from build123d import *

# Parameters (mm, degrees)
BOSS_EXTRUDE1_DEPTH = 40
SKETCH2_R           = 18
SKETCH2_R_2         = 1.5
BOSS_EXTRUDE2_DEPTH = 30.2
SKETCH3_R           = 11
BOSS_EXTRUDE3_DEPTH = 2
BOSS_EXTRUDE4_DEPTH = 20


with BuildPart() as part:
    # Sketch1 → Boss-Extrude1 (new body)
    with BuildSketch(Plane(origin=(0, 0, 0), x_dir=(0, 0, -1), z_dir=(1, 0, 0))):
        Polygon((-21, 15), (-15, 21), (15, 21), (21, 15), (21, -15), (15, -21), (-15, -21), (-21, -15), align=None)
    extrude(amount=BOSS_EXTRUDE1_DEPTH)

    # Sketch2 → Boss-Extrude2 (add)
    with BuildSketch(Plane(origin=(40, 0, 0), x_dir=(0, 0, -1), z_dir=(1, 0, 0))):
        Circle(SKETCH2_R)
        with Locations((-9.899494937, 9.899494937)):
            Circle(SKETCH2_R_2, mode=Mode.SUBTRACT)
        with Locations((9.899494937, 9.899494937)):
            Circle(SKETCH2_R_2, mode=Mode.SUBTRACT)
        with Locations((9.899494937, -9.899494937)):
            Circle(SKETCH2_R_2, mode=Mode.SUBTRACT)
        with Locations((-9.899494937, -9.899494937)):
            Circle(SKETCH2_R_2, mode=Mode.SUBTRACT)
    extrude(amount=BOSS_EXTRUDE2_DEPTH)

    # Sketch3 → Boss-Extrude3 (add)
    with BuildSketch(Plane(origin=(70.2, 0, 0), x_dir=(0, 0, -1), z_dir=(1, 0, 0))):
        Circle(SKETCH3_R)
    extrude(amount=BOSS_EXTRUDE3_DEPTH)

    # Sketch4 → Boss-Extrude4 (add)
    with BuildSketch(Plane(origin=(72.2, 0, 0), x_dir=(0, 0, -1), z_dir=(1, 0, 0))):
        with BuildLine():
            Line((2.645751311, 3), (-2.645751311, 3))
            ThreePointArc((-2.645751311, 3), (0, -4), (2.645751311, 3))
        make_face()
    extrude(amount=BOSS_EXTRUDE4_DEPTH)


solid = part.part
CAD build for the part. Positions are in the model's coordinates, mm. A direction names the side the tool comes from. Coordinates: 2 decimals unless noted, no trailing zeros. Loops run counter-clockwise (first coordinate to the right, second up) from the corner with the lowest first, then second, coordinate; pieces in that order, holes last. Notation, with made-up numbers: (52.5, -34) -> (74.5, -34) arc R33 ccw to (74.5, 5) -> close; hole circle Ø4 at (-30.5, -3). An arc over 180 degrees is marked (long way). One line per item, written item: value.
1. Slice it at A-A on z = 0. Write the cut outline in (x, y).
Answers:
outline: (0, -21) -> (40, -21) -> (40, -18) -> (70.2, -18) -> (70.2, -11) -> (72.2, -11) -> (72.2, -4) -> (92.2, -4) -> (92.2, 3) -> (72.2, 3) -> (72.2, 11) -> (70.2, 11) -> (70.2, 18) -> (40, 18) -> (40, 21) -> (0, 21) -> close
2. Slice it at B-B on y = 0. Write the cut outline in (x, z), and give its area (3 significant figures).
Answers:
outline: (0, -21) -> (40, -21) -> (40, -18) -> (70.2, -18) -> (70.2, -11) -> (72.2, -11) -> (72.2, -4) -> (92.2, -4) -> (92.2, 4) -> (72.2, 4) -> (72.2, 11) -> (70.2, 11) -> (70.2, 18) -> (40, 18) -> (40, 21) -> (0, 21) -> close
area: 2,970 mm^2
3. Pull direction Y, two halves, no side cores. Call faces 4 (the face through (54.889, 17.847, 2.343)), 5 (the face through (40, -10, 10)), 6 (the face through (20, 21, 0)): pulls with the +Y half, pulls with the -Y half, needs draft (parallel to the pull), parting line crosses it, or undercut.
Answers:
face 4: parting line crosses it
face 5: undercut
face 6: pulls with the +Y half
4. Which spindle directions (+Z, -Z, +X, -X, +Y, -Y) get a long thin tool onto all of the face, cutting with end or side? Do faces 1 (the face through (92.2, 0, 0)), 2 (the face through (54.89, -8.89, -8.79)), 3 (the face through (82, 3, 0)). Say none if no direction does.
Answers:
face 1: +Z, -Z, +X, +Y, -Y
face 2: +X
face 3: +Z, -Z, +X, +Y
5. Drill centre lines: line 1 (X direction, y = -16.5, z = 2); line 2 (X direction, y = 9, z = -5); line 3 (Z direction, x = 31, y = 18). Where is each one in solid material? Low to high. Write a range as [from, to].
Answers:
line 1: x = [0, 70.2]
line 2: x = [0, 72.2]
line 3: z = [-18, 18]
6. Slice it at C-C on x = 35. Write the cut outline in (y, z).
Answers:
outline: (-21, -15) -> (-15, -21) -> (15, -21) -> (21, -15) -> (21, 15) -> (15, 21) -> (-15, 21) -> (-21, 15) -> close
7. Slice it at D-D on x = 47. Write the cut outline in (y, z), and give its area (3 significant figures).
Answers:
outline: circle Ø36 at (0, 0); hole circle Ø3 at (-9.9, -9.9); hole circle Ø3 at (-9.9, 9.9); hole circle Ø3 at (9.9, -9.9); hole circle Ø3 at (9.9, 9.9)
area: 990 mm^2
8. Flat gauge pins, fed straight in: P1, Ø2.5, axis at y = -9.5, z = -10, coming from the +X side; P2, Ø10, axis at x = 65.5, z = -9, coming from the +Y side; P3, Ø3, axis at x = 65, z = 10, coming from the -Y side. Where does each tip first touch, or does it go through?
Answers:
P1: stops at x = 70.2
P2: stops at y = 17.55
P3: stops at y = -15.87
